Input: dimensioned drawing with shaded views. Units: mm. Origin: part minimum x, y, z. Round coordinates to 2 decimals unless told otherwise and drop trailing zeros. Loops run counter-clockwise (first coordinate to the right, second up) from the corner with the lowest first, then second, coordinate; pieces in that order, holes last. Notation, with made-up numbers: (-23.75, 55.25) - (6.25, 55.25) arc R9 ccw to (6.25, 67.25) - close; hole circle Ø8 at (16, -28). An arc over 180 degrees is marked (long way). Answer as a JSON object with one key per item and string values. Group by question number.
Item 1: Section B-B (z = 23). Return the cut outline in (x, y).
Item 2: Draft query along X for the marked faces 1, 2, 3 and 4. Return one class per face: released by +X, released by -X, zero draft, split by the parting line, or undercut.
Item 3: Section C-C (y = 25). Return the cut outline in (x, z).
Item 4: Line query: line 1 (Y direction, x = 20, z = 13); line 2 (Y direction, x = 22, z = 3.5); line 3 (Y direction, x = 35, z = 25.5). Output: solid intervals per line, ascending.
Item 5: Section D-D (x = 5). Return the cut outline in (y, z).
Item 6: Section A-A (x = 20). Return the cut outline in (y, z), plus the area to 3 significant figures.
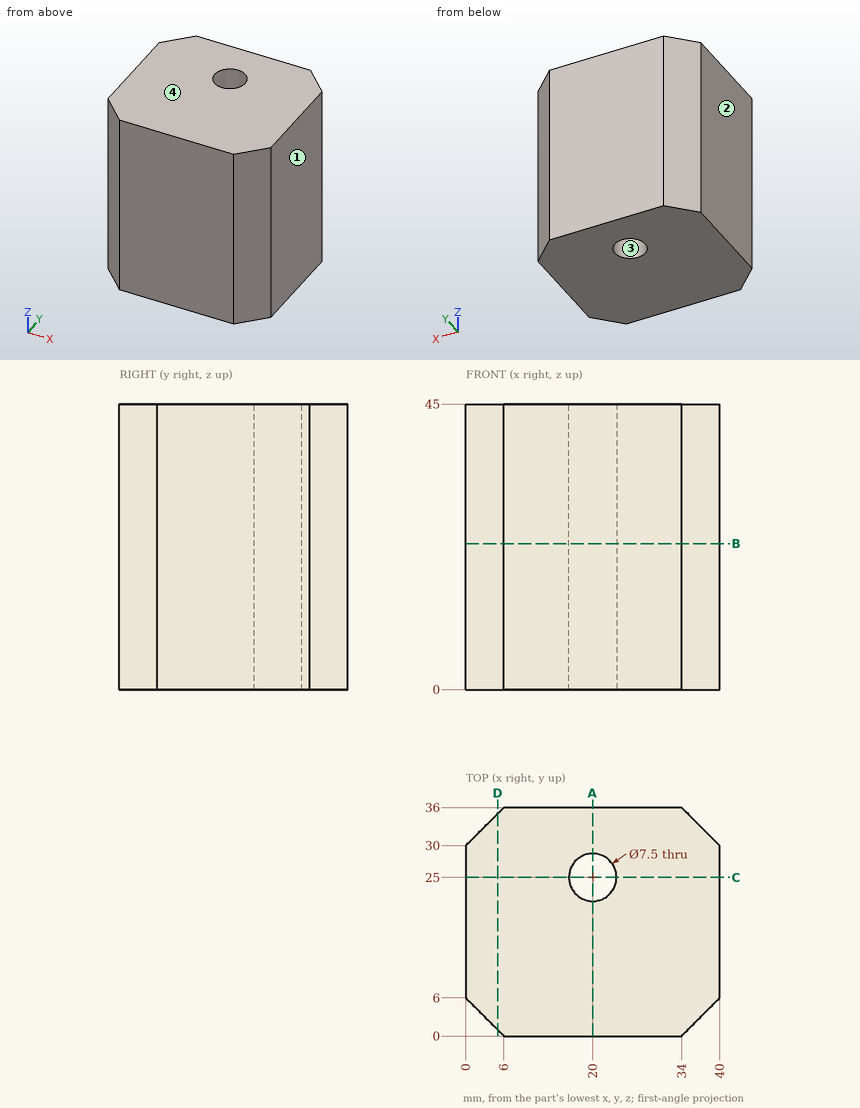
Values:
{
 "1": {"outline": "(0, 6) - (6, 0) - (34, 0) - (40, 6) - (40, 30) - (34, 36) - (6, 36) - (0, 30) - close; hole circle Ø7.5 at (20, 25)"},
 "2": {"face 1": "released by +X", "face 2": "released by -X", "face 3": "undercut", "face 4": "zero draft"},
 "3": {"outline": "(0, 0) - (16.25, 0) - (16.25, 45) - (0, 45) - close; (23.75, 0) - (40, 0) - (40, 45) - (23.75, 45) - close"},
 "4": {"line 1": "y = 0 to 21.25, 28.75 to 36", "line 2": "y = 0 to 21.83, 28.17 to 36", "line 3": "y = 1 to 35"},
 "5": {"outline": "(1, 0) - (35, 0) - (35, 45) - (1, 45) - close"},
 "6": {"outline": "(0, 0) - (21.25, 0) - (21.25, 45) - (0, 45) - close; (28.75, 0) - (36, 0) - (36, 45) - (28.75, 45) - close", "area": "1,280 mm^2"}
}
